Here's the drawing with two shaded views (mm, measured from the low corner). I have some questions. A direction names the side the tool comes from. Round coordinates to 2 decimals unless told otherwise and drop trailing zeros. Write each loop counter-clockwise with the first axis right and the second up, starting at its lowest first coordinate (ties: lowest second). Pieces come first, ordered by that corner, then holes. Notation, with made-up numbers: M 37,-32.75 L 48,-32.75 A17 cw 48,-23.75 Z; hole C -13.75,11.25 d2. An arc over 180 degrees is marked long. Answer as a JSON object with one key per item and string values. Group by question number.
1) Suppose I cut it at D-D, the plane y = 4.75. Write out the boundary of the cut face in (x, z) (3 decimals), and give its area (3 significant figures).
2) Suppose I cut it at B-B, the plane x = 1.75. Write out the boundary of the cut face in (y, z).
3) On a 3-axis mill with a long thin cutter (end or side, diameter ignored), from which of +Z, -Z, +X, -X, +Y, -Y can I reach the whole of each face in a straight line? I mean the marked faces 1 and 2. Say none if no direction works.
4) I'm going to push flat-ended pins straight in: pin 1 Ø1 at (x, y) = (10.5, 4) entering from -Z; pin 2 Ø0.6 at (x, y) = (8.5, 6) entering from +Z; pin 3 Ø2 at (y, z) = (2, 3) entering from +X (3 decimals); pin 4 Ø1.6 at (x, z) = (9.5, 3.5) entering from -Y. Where does each tip first touch, or does it pass through?
5) Suppose I cut it at C-C, the plane z = 4.15. Write out the boundary of the cut face in (x, y).
6) Please list where these lines run through material, in increasing order: L1, parallel to X at y = 2.5, z = 2.75; L2, parallel to X at y = 4, z = 3.2; L3, parallel to Y at x = 5.75, z = 2.2. Write a range as [from, to].
7) Suppose I cut it at A-A, the plane z = 3.15. Write out the boundary of the cut face in (x, y).
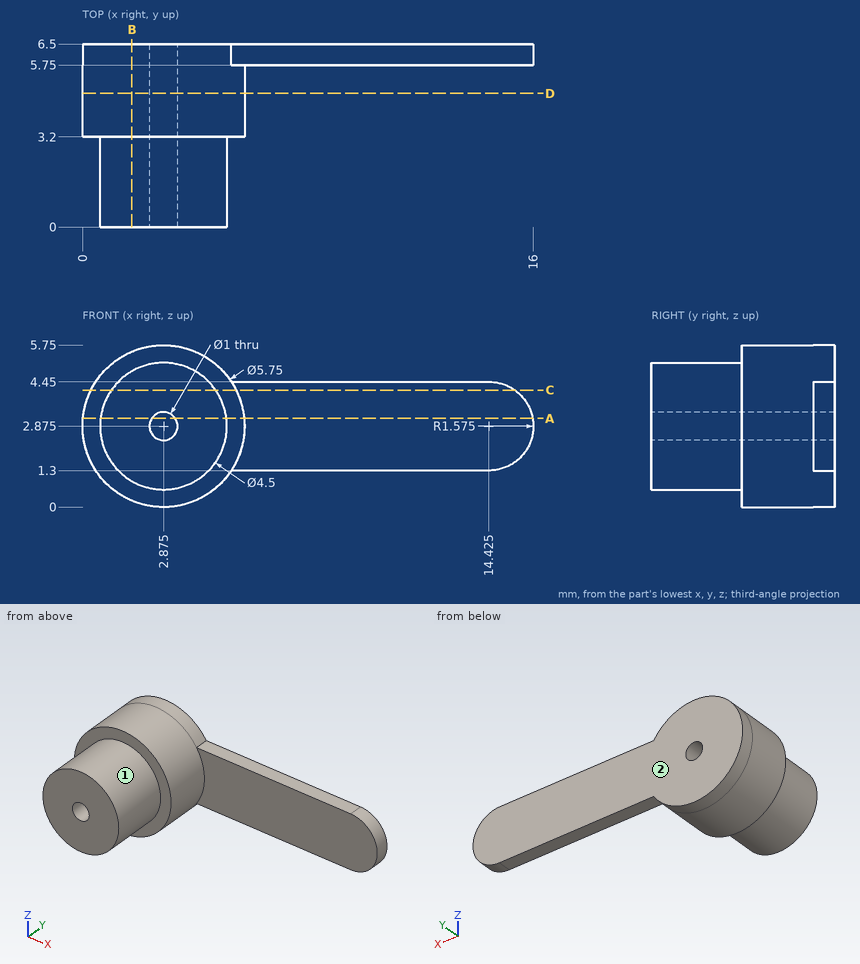
Results:
{
 "1": {"outline": "C 2.875,2.875 d5.75; hole C 2.875,2.875 d1", "area": "25.2 mm^2"},
 "2": {"outline": "M 0,0.93 L 3.2,0.93 L 3.2,0.23 L 6.5,0.23 L 6.5,5.52 L 3.2,5.52 L 3.2,4.82 L 0,4.82 Z"},
 "3": {"face 1": "-Y", "face 2": "+Z, -Z, +X, -X, +Y"},
 "4": {"pin 1": "through", "pin 2": "z = 4.45", "pin 3": "x = 5.125", "pin 4": "y = 5.75"},
 "5": {"outline": "M 0.3,3.2 L 1.02,3.2 L 1.02,0 L 4.73,0 L 4.73,3.2 L 5.45,3.2 L 5.45,5.75 L 15.35,5.75 L 15.35,6.5 L 0.3,6.5 Z"},
 "6": {"L1": "[0.63, 2.39], [3.36, 5.12]", "L2": "[0.02, 2.5], [3.25, 5.73]", "L3": "[5.75, 6.5]"},
 "7": {"outline": "M 0.01,3.2 L 0.64,3.2 L 0.64,0 L 2.46,0 L 2.46,6.5 L 0.01,6.5 Z; M 3.29,0 L 5.11,0 L 5.11,3.2 L 5.74,3.2 L 5.74,5.75 L 15.98,5.75 L 15.98,6.5 L 3.29,6.5 Z"}
}
